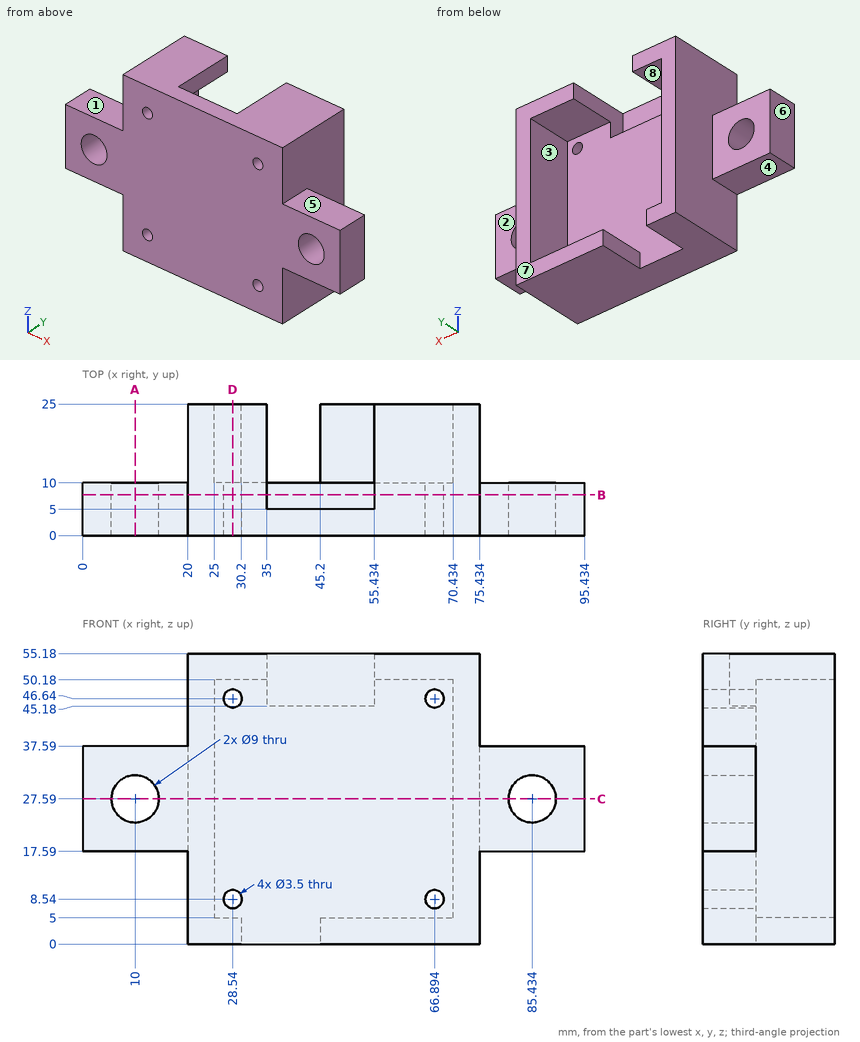
Drawing for the job (mm, zero at the part's lowest x, y, z). A direction names the side the tool comes from. Give positions to 0.01 mm unless a question says otherwise; leave off trailing zeros. Order: outer loops, then holes, each group sorted by start corner. A loop starts at its lowest first (then second) coordinate and runs counter-clockwise, first axis right, second up. Notation, with made-up numbers: M 80.5,-4 L 119.5,-4 A25 cw 119.5,29 Z; hole C 3,31.5 d3. An arc over 180 degrees is marked long. Put each result on its own line as item: value.
Item 1: Slice it at C-C, the plane z = 27.59. Write the cut outline in (x, y), plus the area to 3 significant figures.
From the geometry:
outline: M 0,0 L 5.5,0 L 5.5,10 L 0,10 Z; M 14.5,0 L 80.93,0 L 80.93,10 L 75.43,10 L 75.43,25 L 70.43,25 L 70.43,10 L 25,10 L 25,25 L 20,25 L 20,10 L 14.5,10 Z; M 89.93,0 L 95.43,0 L 95.43,10 L 89.93,10 Z
area: 924 mm2
Item 2: Probe line 1 (X direction, y = 7.5, z = 8.54); line 2 (X direction, y = 2.25, z = 27.59); line 3 (Z direction, x = 28.54, y = 5.25). List the from-to ranges inside material, lowest first. Write a range as [from, to].
From the geometry:
line 1: x = [20, 26.79], [30.29, 65.14], [68.64, 75.43]
line 2: x = [0, 5.5], [14.5, 80.93], [89.93, 95.43]
line 3: z = [0, 6.79], [10.29, 44.89], [48.39, 55.18]
Item 3: 3-axis set-ups, long thin cutter, end or side, ignore diameter. For the marked faces 1, 2, 3, 4 and 5: which of +Z, -Z, +X, -X, +Y, -Y reach the whole face in a straight line?
From the geometry:
face 1: +Z, -X, +Y, -Y
face 2: +Z, -Z, +X, +Y
face 3: +Y
face 4: -Z, -X, +Y, -Y
face 5: +Z, +X, +Y, -Y
Item 4: Two-plate mould, pull along X, no slides. Class the marked faces 6, 7 and 8: +X half, -X half, draft (parallel to the pull), parting line (faces both ways), or undercut.
From the geometry:
face 6: -X half
face 7: draft
face 8: undercut
Item 5: Slice it at D-D, the plane x = 28.54. Write the cut outline in (y, z), plus the area to 3 significant figures.
From the geometry:
outline: M 0,0 L 25,0 L 25,5 L 10,5 L 10,6.79 L 0,6.79 Z; M 0,10.29 L 10,10.29 L 10,44.89 L 0,44.89 Z; M 0,48.39 L 10,48.39 L 10,50.18 L 25,50.18 L 25,55.18 L 0,55.18 Z
area: 632 mm2
Item 6: Slice it at B-B, the plane y = 7.75. Write the cut outline in (x, z).
From the geometry:
outline: M 0,17.59 L 20,17.59 L 20,0 L 75.43,0 L 75.43,17.59 L 95.43,17.59 L 95.43,37.59 L 75.43,37.59 L 75.43,55.18 L 55.43,55.18 L 55.43,45.18 L 35,45.18 L 35,55.18 L 20,55.18 L 20,37.59 L 0,37.59 Z; hole C 10,27.59 d9; hole C 28.54,8.54 d3.5; hole C 28.54,46.64 d3.5; hole C 66.89,8.54 d3.5; hole C 66.89,46.64 d3.5; hole C 85.43,27.59 d9
Item 7: Flat gauge pins, fed straight in: pin 1 Ø10.5 at (x, z) = (85.434, 27.59) entering from +Y; pin 2 Ø5.5 at (x, y) = (47.5, 8.5) entering from +Z; pin 3 Ø8 at (y, z) = (19, 51) entering from -X; pin 4 Ø8 at (x, z) = (10, 27.59) entering from -Y. Where does each tip first touch, or does it go through?
From the geometry:
pin 1: stops at y = 10
pin 2: stops at z = 45.18
pin 3: stops at x = 20
pin 4: passes through
Item 8: Slice it at A-A, the plane x = 10. Write the cut outline in (y, z), plus the area to 3 significant figures.
From the geometry:
outline: M 0,17.59 L 10,17.59 L 10,23.09 L 0,23.09 Z; M 0,32.09 L 10,32.09 L 10,37.59 L 0,37.59 Z
area: 110 mm2
